Geometry check sheet. Reference: drawing and pictorial views, mm from the part's lowest x, y, z. Round coordinates to 2 decimals unless told otherwise and drop trailing zeros. Order: outer loops, then holes, each group sorted by start corner. A loop starts at its lowest first (then second) coordinate and runs counter-clockwise, first axis right, second up.
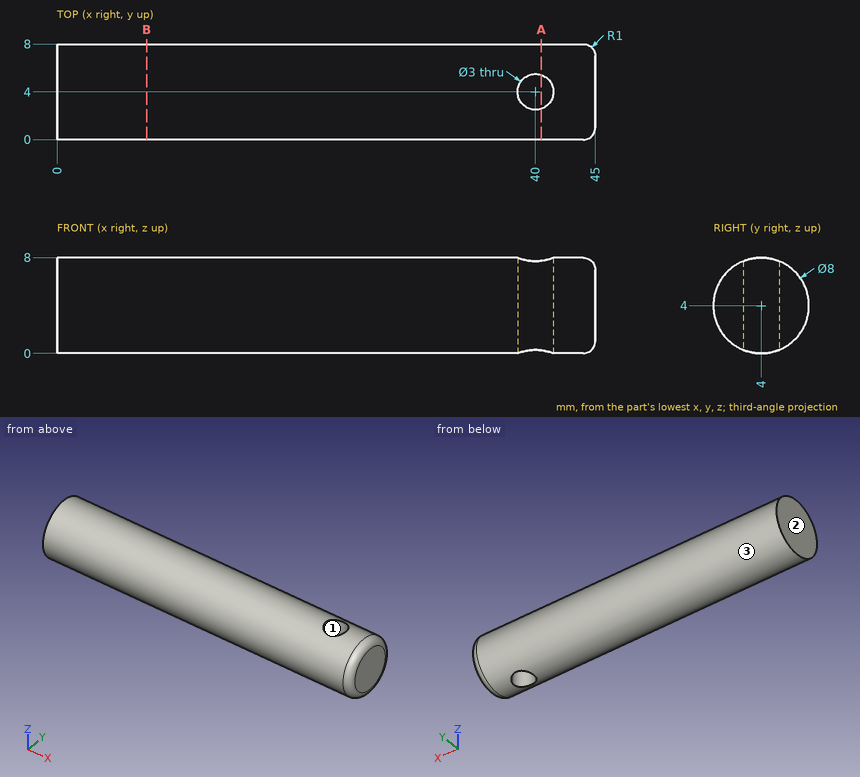
1) Scan lines: probe 1 along X at (y, z) = (4, 3.25); probe 2 along X at (y, z) = (3.5, 1.25); probe 3 along Y at (x, z) = (14.5, 1.5). Record each from-to range of solid material in increasing order.
2) Sectioned sample at A-A on x = 40.5. Record the cut outline in (y, z), then the cut area to 3 significant figures.
3) Sectioned sample at B-B on x = 7.5. Record the cut outline in (y, z).
4) Go/stop test with flat-tipped pins: pin 1 Ø3 at (x, y) = (33, 1.5) entering from -Z; pin 2 Ø4 at (x, z) = (20, 1.5) entering from -Y. Record where each tip stops, or that it passes through.
5) Draft check along Y on the marked faces 1, 2 and 3. Enter one of: released by +Y, released by -Y, zero draft, split by the parting line, or undercut.
Returned:
1. probe 1: x = 0 to 38.5, 41.5 to 45
1. probe 2: x = 0 to 38.59, 41.41 to 45
1. probe 3: y = 0.88 to 7.12
2. outline: (2.59, 0.26) - (2.59, 7.74) arc R4 ccw to start; (5.41, 0.26) arc R4 ccw to (5.41, 7.74) - close
2. area: 28.1 mm2
3. outline: circle Ø8 at (4, 4)
4. pin 1: stops at z = 0.13
4. pin 2: stops at y = 0.03
5. face 1: undercut
5. face 2: zero draft
5. face 3: split by the parting line
